Check sheet for the modelled part. Datum: model origin and axes. Units: mm. A direction names the side the tool comes from. Give positions to 0.01 mm unless a question says otherwise; leave off trailing zeros. Write each loop counter-clockwise with the first axis right and the second up, starting at its lowest first coordinate (ties: lowest second). Pieces come first, ordered by that corner, then holes. Notation, with made-up numbers: M 81,-26 L 108,-26 A15 ccw 108,3 Z; hole C 9.25,38.5 d9. An arc over 180 degrees is marked long. Use CSV: the item, a comma, the result in double quotes. Start each with the question number.
1. Cross-section at D-D, the plane x = -26. Enter the section's corners in (y, z).
2. Depth check by flat-ended pin: P1, Ø1, axis at x = 2.5, y = -4, coming from the +Z side; P2, Ø7.5, axis at x = 20, y = -18, coming from the +Z side. Enter the tip coordinate at first touch or a pass-through.
3. Cross-section at C-C, the plane y = -12.7. Enter the section's corners in (x, z) (3 decimals), and give its area (3 significant figures).
4. Access from +Z, -Z, +X, -X, +Y, -Y to the whole of each face (thin tool, end or side, straight path). Record for faces 4 (the face through (41.471, -13, 2)), 5 (the face through (-42.604, -12.784, -9.371)), 6 (the face through (23, -13, 14.728)), 7 (the face through (-30.26, -12.77, 15.73)).
5. Cross-section at B-B, the plane x = 32. Enter the section's corners in (y, z), and give its area (3 significant figures).
6. Scan lines: line 1 (Y direction, x = -33.5, z = 7.5); line 2 (Y direction, x = -49, z = 0); line 3 (X direction, y = -12.7, z = 28.5) (3 decimals). Record each from-to range of solid material in increasing order.
7. Cross-section at A-A, the plane z = 21. Enter the section's corners in (x, y).
8. Mould release check, pull along Y, two halves, no side actions. Record for faces 1 (the face through (-21, -25.4, 9)), 2 (the face through (-41, -13, 40.128)), 3 (the face through (-26.962, -12.771, 8.254)): +Y half, -Y half, draft (parallel to the pull), parting line (faces both ways), or undercut.
from build123d import *

# Parameters (mm, degrees)
F1_DEPTH = 25.4
F2_R     = 4.826
F3_DEPTH = 50.801
F4_W     = 7.62
F4_H     = 10.16
F5_DEPTH = 62.862793


with BuildPart() as f1:
    # F0 (on Front) → F1 (new body)
    with BuildSketch(Plane.XZ):
        Polygon((-22.029007, 40.128093), (-60.129007, 40.128093), (-60.129007, -10.671907), (41.470993, -10.671907), (41.470993, 14.728093), (3.370993, 14.728093), align=None)
    extrude(amount=F1_DEPTH)

    # F2 (on face) → F3 (cut, through all)
    with BuildSketch(Plane.XY.offset(40.128093)):
        with Locations((-47.429007, -12.7)):
            Circle(F2_R)
        with Locations((28.770993, -12.7)):
            Circle(F2_R)
    extrude(amount=-F3_DEPTH, mode=Mode.SUBTRACT)

    # F4 (on face) → F5 (cut, through all)
    with BuildSketch(Plane(origin=(9.049543, 0, 9.049543), x_dir=(0.707107, 0, -0.707107), z_dir=(0.707107, 0, 0.707107))):
        with Locations((-28.711707, -12.7)):
            Rectangle(F4_W, F4_H)
    extrude(amount=-F5_DEPTH, mode=Mode.SUBTRACT)


solid = f1.part
Worked answers:
1,outline,"M -25.4,-10.67 L 0,-10.67 L 0,40.13 L -25.4,40.13 Z; hole M -17.78,9.22 L -7.62,9.22 L -7.62,19.99 L -17.78,19.99 Z"
2,P1,"stops at z = 16.1"
2,P2,"stops at z = 14.73"
3,outline,"M -60.129,-10.672 L -56.665,-10.672 L -52.255,-6.262 L -52.255,40.128 L -60.129,40.128 Z; M -42.603,-10.672 L 23.945,-10.672 L 23.945,14.728 L 3.371,14.728 L -8.559,26.658 L -42.603,-7.387 Z; M -42.603,3.39 L -13.947,32.046 L -22.029,40.128 L -42.603,40.128 Z; M 33.597,-10.672 L 41.471,-10.672 L 41.471,14.728 L 33.597,14.728 Z"
3,area,"2,790 mm^2"
4,face 4,"+Z, -Z, +X, +Y, -Y"
4,face 5,"+Z, -Z"
4,face 6,"+Z, +X, +Y, -Y"
4,face 7,"none"
5,outline,"M -25.4,-10.67 L -16.29,-10.67 L -16.29,14.73 L -25.4,14.73 Z; M -9.11,-10.67 L 0,-10.67 L 0,14.73 L -9.11,14.73 Z"
5,area,"463 mm^2"
6,line 1,"y = -25.4 to -17.78, -7.62 to 0"
6,line 2,"y = -25.4 to -17.26, -8.14 to 0"
6,line 3,"x = -60.129 to -52.255, -42.603 to -17.493"
7,outline,"M -60.13,-25.4 L -2.9,-25.4 L -2.9,0 L -60.13,0 Z; hole C -47.43,-12.7 d9.65; hole M -24.99,-17.78 L -14.22,-17.78 L -14.22,-7.62 L -24.99,-7.62 Z"
8,face 1,"-Y half"
8,face 2,"draft"
8,face 3,"undercut"
